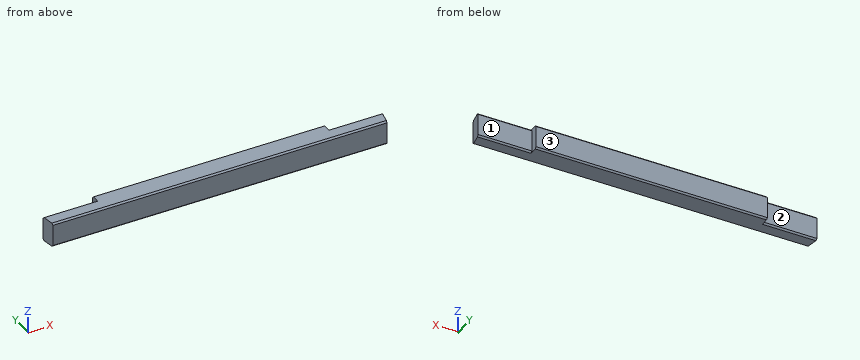
Autodesk Inventor part; units mm, degrees
ref_plane "YZ Plane" through (0, 0, 0) normal (1, 0, 0) x (0, 1, 0)
ref_plane "XZ Plane" through (0, 0, 0) normal (0, 1, 0) x (-1, 0, 0)
ref_plane "XY Plane" through (0, 0, 0) normal (0, 0, 1) x (1, 0, 0)
sketch "Sketch1" plane through (0, 0, 0) normal (0, 0, 1) x (1, 0, 0)
  line L0 (-357.2554, -61.8782) -> (-427.6081, -61.8782) construction
  line L1 (-357.2554, -61.8782) -> (-357.2554, -55.8782) construction
  line L2 (-405.0222, -45.9997) -> (-425.3346, 69.1978) construction
  line L3 (-419.5247, 76.1218) -> (-425.3346, 69.1978) construction
  line L4 (-408.3518, 76.1218) -> (-408.3518, 82.1218) construction
  line L5 (-450.7203, 69.1978) -> (-427.6081, -61.8782) construction
  line L6 (13.9045, -61.8782) -> (-56.4482, -61.8782) construction
  line L7 (13.9045, -61.8782) -> (37.0167, 69.1978) construction
  line L8 (-5.3518, 82.1218) -> (-5.3518, 76.1218) construction
  line L9 (11.631, 69.1978) -> (5.8211, 76.1218) construction
  line L10 (11.631, 69.1978) -> (-8.6814, -45.9997) construction
  line L11 (-56.4482, -55.8782) -> (-56.4482, -61.8782) construction
  line L12 (13.5518, -63.8782) -> (13.9045, -61.8782) construction
  line L13 (13.9045, -61.8782) -> (-56.4482, -61.8782) construction
  line L14 (-56.4482, -61.8782) -> (-56.4482, -63.8782) construction
  line L15 (-56.4482, -63.8782) -> (13.5518, -63.8782) construction
  line L16 (-357.2554, -63.8782) -> (-357.2554, -61.8782) construction
  line L17 (-357.2554, -61.8782) -> (-427.6081, -61.8782) construction
  line L18 (-427.6081, -61.8782) -> (-427.2554, -63.8782) construction
  line L19 (-427.2554, -63.8782) -> (-357.2554, -63.8782) construction
  line L20 (-347.2554, -53.8782) -> (-66.4482, -53.8782)
  line L21 (-56.4482, -63.8782) -> (13.5518, -63.8782)
  line L22 (13.5518, -63.8782) -> (10.3779, -81.8782)
  line L23 (10.3779, -81.8782) -> (-424.0815, -81.8782)
  line L24 (-424.0815, -81.8782) -> (-427.2554, -63.8782)
  line L25 (-427.2554, -63.8782) -> (-357.2554, -63.8782)
  line L26 (45.2684, 76.1218) -> (37.0167, 69.1978)
  line L27 (94.6482, 76.1218) -> (94.6482, 82.1218)
  line L28 (-508.3518, 82.1218) -> (-508.3518, 76.1218)
  line L29 (-450.7203, 69.1978) -> (-458.972, 76.1218)
  line L30 (-5.3518, 82.1218) -> (94.6482, 82.1218)
  line L31 (-508.3518, 82.1218) -> (-408.3518, 82.1218)
  line L32 (-56.4482, -55.8782) -> (-20.4541, -55.8782)
  line L33 (94.6482, 76.1218) -> (45.2684, 76.1218)
  line L34 (5.8211, 76.1218) -> (-5.3518, 76.1218)
  line L35 (-20.4541, -55.8782) -> (-8.6814, -45.9997)
  line L36 (-405.0222, -45.9997) -> (-393.2495, -55.8782)
  line L37 (-408.3518, 76.1218) -> (-419.5247, 76.1218)
  line L38 (-458.972, 76.1218) -> (-508.3518, 76.1218)
  line L39 (-393.2495, -55.8782) -> (-357.2554, -55.8782)
  line L40 (-66.4482, -53.8782) -> (-56.4482, -53.8782)
  line L41 (-56.4482, -53.8782) -> (-56.4482, -63.8782)
  line L42 (-357.2554, -63.8782) -> (-357.2554, -53.8782)
  line L43 (-357.2554, -53.8782) -> (-347.2554, -53.8782)
  point P0 (0, 0)
  dimension "d0" = 28
extrude "Extrusion1" add sketch "Sketch1" against normal blind 32
chamfer "Chamfer1" distance 2 angle 45 8 edges at (-392.2554, -63.8782, 0) (-392.2554, -63.8782, -32) (-206.8518, -81.8782, -32) (-206.8518, -81.8782, 0) (-21.4482, -63.8782, 0) (-21.4482, -63.8782, -32) (-206.8518, -53.8782, 0) (-206.8518, -53.8782, -32)
properties part number "DNW_CON_V2" material "Wood (Birch)"
Geometry check sheet. Reference: the model listing, model coordinates, mm. Face numbers are marked on the shaded views. A direction names the side the tool comes from. Round coordinates to 2 decimals unless told otherwise and drop trailing zeros. Loops run counter-clockwise (first coordinate to the right, second up) from the corner with the lowest first, then second, coordinate; pieces in that order, holes last. Notation, with made-up numbers: (51, 46) - (62, 46) arc R23 ccw to (62, 58) - close; hole circle Ø8 at (11.25, 17.5). An arc over 180 degrees is marked (long way). One line per question, with ' | ' between items. Start each with the question number.
1. Cross-section at B-B on z = -26. Record the cut outline in (x, y), then the cut area to 3 significant figures.
2. Depth check by flat-ended pin: pin 1 (9.5 mm diameter, centred on y = -61, z = -11.5, fed in from -X); pin 2 (5 mm diameter, centred on y = -73, z = -27.5, fed in from -X); pin 3 (4 mm diameter, centred on y = -69, z = -25.5, fed in from +X); pin 4 (3.5 mm diameter, centred on y = -61.5, z = -14.5, fed in from +X). Enter the tip coordinate at first touch or a pass-through.
3. Cross-section at C-C on y = -60.25. Record the cut outline in (x, z), then the cut area to 3 significant figures.
4. Scan lines: line 1 (Y direction, x = -52.5, z = -22); line 2 (X direction, y = -62.5, z = -24.5); line 3 (Z direction, x = -79, y = -80.5). Record each from-to range of solid material in increasing order. Write a range as [from, to].
5. Cross-section at A-A on x = -34. Record the cut outline in (y, z).
6. Tool access check on the marked faces 1, 2 and 3. Record the directions out of +Z, -Z, +X, -X, +Y, -Y that give a thin tool (end or side, any length) a straight path to the whole face; none if there is none.
Taken from the geometry:
1) outline: (-427.26, -63.88) - (-424.08, -81.88) - (10.38, -81.88) - (13.55, -63.88) - (-56.45, -63.88) - (-56.45, -53.88) - (-357.26, -53.88) - (-357.26, -63.88) - close | area: 10,900 mm²
2) pin 1: x = -427.26 | pin 2: x = -426.09 | pin 3: x = 13 | pin 4: x = -56.45
3) outline: (-357.26, -32) - (-56.45, -32) - (-56.45, 0) - (-357.26, 0) - close | area: 9,630 mm²
4) line 1: [-81.88, -63.88] | line 2: [-357.26, -56.45] | line 3: [-31.38, -0.62]
5) outline: (-81.88, -30) - (-79.88, -32) - (-65.88, -32) - (-63.88, -30) - (-63.88, -2) - (-65.88, 0) - (-79.88, 0) - (-81.88, -2) - close
6) face 1: +Z, -Z, +X, +Y | face 2: +Z, -Z, -X, +Y | face 3: +Z, -Z, +X, -X, +Y
